Verification items for the finished model (mm, model axes). Give positions to 0.01 mm unless a question says otherwise; leave off trailing zeros. Loops run counter-clockwise (first coordinate to the right, second up) from the corner with the lowest first, then second, coordinate; pieces in that order, holes last. Notation, with made-up numbers: (-13.5, 45.25) - (30.5, 45.25) arc R24 ccw to (30.5, 60.25) - close; hole circle Ø2 at (84, 33). An arc over 180 degrees is marked (long way). One line per question, with ' | ' between items. Start each with the question number.
1. Section check B-B, the plane z = -0.35. Enter the section's corners in (x, y), then the cut area to 3 significant figures.
2. Thickness scan on line 1 along Y through (x, z) = (10, -0.55); line 2 along X through (y, z) = (59.5, -1.8). Record the ranges inside material, lowest first. Write a range as from..to.
3. Depth check by flat-ended pin: pin 1 Ø1 at (y, z) = (44.5, -1) entering from +X; pin 2 Ø4.5 at (x, y) = (10, 25) entering from +Z. Enter the tip coordinate at first touch or a pass-through.
4. Section check D-D, the plane x = 25. Enter the section's corners in (y, z).
5. Section check A-A, the plane x = 10. Enter the section's corners in (y, z).
Autodesk Inventor part; units mm, degrees
ref_plane "YZ Plane" through (0, 0, 0) normal (1, 0, 0) x (0, 1, 0)
ref_plane "XZ Plane" through (0, 0, 0) normal (0, 1, 0) x (-1, 0, 0)
ref_plane "XY Plane" through (0, 0, 0) normal (0, 0, 1) x (1, 0, 0)
sketch "Эскиз1" plane through (0, 0, 0) normal (0, 0, 1) x (1, 0, 0)
  line L0 (0, 0) -> (75, 0)
  line L1 (20, 20) -> (20, 75)
  line L2 (0, 75) -> (0, 0)
  line L3 (20, 20) -> (75, 20)
  circle A0 centre (10, 131.9318) radius 2.5
  circle A1 centre (10, 65) radius 2.5
  circle A2 centre (10, 25) radius 2.5
  circle A3 centre (25, 10) radius 2.5
  circle A4 centre (65, 10) radius 2.5
  line L4 (0, 75) -> (20, 75)
  line L5 (75, 0) -> (75, 20)
  point P0 (10, 75)
  point P1 (75, 10)
  dimension "d5" = 5
  dimension "d11" = 20
  dimension "d12" = 20
  dimension "d13" = 75
  dimension "d14" = 10
  dimension "d15" = 40
  dimension "d16" = 10
  dimension "d17" = 40
extrude "Выдавливание1" add sketch "Эскиз1" against normal blind 2 contours L2 L4 L1 L3 L5 L0
equation "\"d16\" = d14"
equation "\"d17\" = d15"
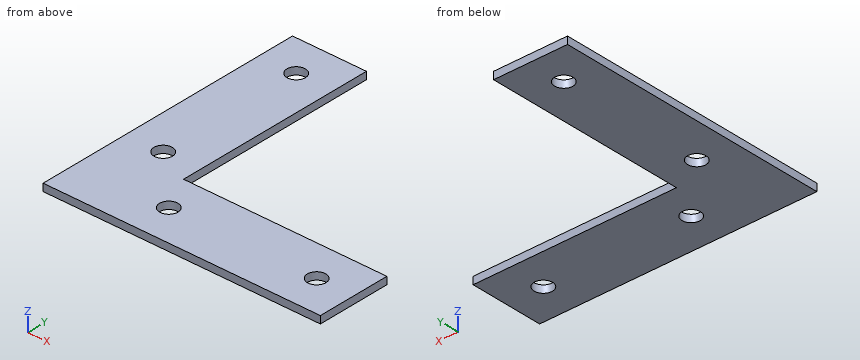
Results list:
1) outline: (0, 0) - (75, 0) - (75, 20) - (20, 20) - (20, 75) - (0, 75) - close; hole circle Ø5 at (10, 25); hole circle Ø5 at (10, 65); hole circle Ø5 at (25, 10); hole circle Ø5 at (65, 10) | area: 2,520 mm²
2) line 1: 0..22.5, 27.5..62.5, 67.5..75 | line 2: 0..20
3) pin 1: x = 20 | pin 2: through
4) outline: (0, -2) - (7.5, -2) - (7.5, 0) - (0, 0) - close; (12.5, -2) - (20, -2) - (20, 0) - (12.5, 0) - close
5) outline: (0, -2) - (22.5, -2) - (22.5, 0) - (0, 0) - close; (27.5, -2) - (62.5, -2) - (62.5, 0) - (27.5, 0) - close; (67.5, -2) - (75, -2) - (75, 0) - (67.5, 0) - close
